Model file for the job. Use its own axes, mm. A direction names the side the tool comes from. Coordinates: 2 decimals unless noted, no trailing zeros. Loops run counter-clockwise (first coordinate to the right, second up) from the corner with the lowest first, then second, coordinate; pieces in that order, holes last. Notation, with made-up numbers: M -16,36.5 L 40,36.5 A12 ccw 40,50.5 Z; hole C 18,-25.75 d1. An arc over 180 degrees is marked long. One line per question, with ' | ' between items. Start each with the question number.
```python
from build123d import *

# Parameters (mm, degrees)
BOSS_EXTRUDE1_DEPTH = 10
SKETCH3_W           = 20
SKETCH3_H           = 10
CUT_EXTRUDE2_DEPTH  = 27.5
SKETCH4_R           = 2.5
BOSS_EXTRUDE2_DEPTH = 10
SKETCH5_R           = 1.25
CUT_EXTRUDE4_DEPTH  = 10
SKETCH6_R           = 2.5
CUT_EXTRUDE5_DEPTH  = 1.25


with BuildPart() as part:
    # Sketch1 → Boss-Extrude1 (new body, symmetric)
    with BuildSketch(Plane.XY):
        with BuildLine():
            Line((-10, 22.5), (-10, 0))
            Line((-10, 0), (10, 0))
            Line((10, 0), (10, 22.5))
            ThreePointArc((10, 22.5), (0, 32.5), (-10, 22.5))
        make_face()
    extrude(amount=BOSS_EXTRUDE1_DEPTH, both=True)

    # Sketch3 → Cut-Extrude2 (cut)
    with BuildSketch(Plane(origin=(0, 32.5, 0), x_dir=(1, 0, 0), z_dir=(0, 1, 0))):
        Rectangle(SKETCH3_W, SKETCH3_H)
    extrude(amount=-CUT_EXTRUDE2_DEPTH, mode=Mode.SUBTRACT)

    # Sketch4 → Boss-Extrude2 (add)
    with BuildSketch(Plane(origin=(0, 0, 5), x_dir=(-1, 0, 0), z_dir=(0, 0, -1))):
        with Locations((0, 24.5)):
            Circle(SKETCH4_R)
    extrude(amount=BOSS_EXTRUDE2_DEPTH)

    # Sketch5 → Cut-Extrude4 (cut)
    with BuildSketch(Plane(origin=(0, 5, 0), x_dir=(1, 0, 0), z_dir=(0, 1, 0))):
        Circle(SKETCH5_R)
    extrude(amount=-CUT_EXTRUDE4_DEPTH, mode=Mode.SUBTRACT)

    # Sketch6 → Cut-Extrude5 (cut)
    with BuildSketch(Plane(origin=(0, 5, 0), x_dir=(1, 0, 0), z_dir=(0, 1, 0))):
        Circle(SKETCH6_R)
    extrude(amount=-CUT_EXTRUDE5_DEPTH, mode=Mode.SUBTRACT)


solid = part.part
```
(1) 3-axis set-ups, long thin cutter, end or side, ignore diameter. For faces 1 (the face through (-2.4, 5, -1.2)), 2 (the face through (0, 16, -10)), 3 (the face through (2, 0, 0)), 4 (the face through (0, 27, 0)), 5 (the face through (-0.27, 1.9, 1.22)): which of +Z, -Z, +X, -X, +Y, -Y reach the whole face in a straight line?
(2) Drill centre lines: line 1 (Z direction, x = -3.25, y = 5.5); line 2 (X direction, y = 2.8, z = 0). Where is each one in solid material? Low to high. Write a range as [from, to].
(3) Pin check, flat tips, straight feed: P1, Ø3, axis at x = 0, z = 0, coming from the -Y side; P2, Ø1, axis at x = -2, z = -3.5, coming from the +Y side; P3, Ø2.5, axis at x = -1, z = -0.5, coming from the +Y side; P4, Ø1, axis at x = -2, z = 5, coming from the +Y side. Stop position of each tip, or through.
(4) Band-saw the part on C-C on x = 0. Write the cut outline in (y, z), then the cut area to 3 significant figures.
(5) Band-saw the part on A-A on z = 3.25. Write the cut outline in (x, y).
(6) Band-saw the part on D-D on y = 28. Write the cut outline in (x, z), then the cut area to 3 significant figures.
(7) Band-saw the part on B-B on y = 17.5. Write the cut outline in (x, z), then the cut area to 3 significant figures.
(8) Two-plate mould, pull along Y, no slides. Class faces 6 (the face through (0, 19, -5)), 7 (the face through (10, 4, 0)), 8 (the face through (0.2, 32.5, -7.5)), 9 (the face through (-0.54, 4.38, 2.44)): pulls with the +Y half, pulls with the -Y half, needs draft (parallel to the pull), parting line crosses it, or undercut.
Computed values:
1) face 1: +X, -X | face 2: -Z, +X, -X, +Y, -Y | face 3: +Z, -Z, +X, -X, -Y | face 4: none | face 5: -Y
2) line 1: [-10, -5], [5, 10] | line 2: [-10, -1.25], [1.25, 10]
3) P1: y = 0 | P2: y = 26.5 | P3: y = 27 | P4: y = 32.39
4) outline: M 0,-10 L 32.5,-10 L 32.5,-5 L 27,-5 L 27,5 L 32.5,5 L 32.5,10 L 0,10 L 0,1.25 L 3.75,1.25 L 3.75,2.5 L 5,2.5 L 5,5 L 22,5 L 22,-5 L 5,-5 L 5,-2.5 L 3.75,-2.5 L 3.75,-1.25 L 0,-1.25 Z | area: 409 mm^2
5) outline: M -10,0 L 10,0 L 10,5 L -10,5 Z; C 0,24.5 d5
6) outline: M -8.35,-10 L 8.35,-10 L 8.35,-5 L -8.35,-5 Z; M -8.35,5 L 8.35,5 L 8.35,10 L -8.35,10 Z | area: 167 mm^2
7) outline: M -10,-10 L 10,-10 L 10,-5 L -10,-5 Z; M -10,5 L 10,5 L 10,10 L -10,10 Z | area: 200 mm^2
8) face 6: undercut | face 7: needs draft | face 8: pulls with the +Y half | face 9: undercut
